Can you work these out from the model? Positions are in its coordinate system, mm. A direction names the side the tool comes from. Coordinates: 2 decimals unless noted, no trailing zeros. Loops run counter-clockwise (first coordinate to the right, second up) from the corner with the lowest first, then second, coordinate; pieces in that order, holes last. Notation, with made-up numbers: (42, 87.5) -> (54, 87.5) arc R14 ccw to (54, 96.5) -> close; hole circle Ø2 at (5.5, 39.25). An arc over 180 degrees is marked (long way). Put each result on its own line as item: value. Start each with the question number.
Item 1: Please list where these lines run through material, in increasing order: L1, parallel to Z at x = 25.09, y = 16.85; L2, parallel to Z at x = 8, y = 21; L3, parallel to X at y = 2, z = -4.5. Write a range as from..to.
Item 2: If we section it at C-C on x = 10.75: Please give me the cut outline in (y, z), plus the area to 3 significant figures.
Item 3: For faces 1 (the flat face through (23.9, 16, -6.2)), 2 (the flat face through (0, 8, -6)), 3 (the cylindrical face through (8.1, 24.5, -6.2)), which set-ups out of +Z, -Z, +X, -X, +Y, -Y let a thin tool reach every point of the face, with its end or its side?
Item 4: If we section it at D-D on z = -4.5: Please give me the cut outline in (x, y), plus the area to 3 significant figures.
Item 5: We'd pull the mould along Z, two halves only. Please class faces 4 (the cylindrical face through (-1.74, 17.27, -6.31)), 5 (the flat face through (27, 17, -5.862)), 6 (the flat face through (27.25, 17, -9)), 7 (the cylindrical face through (14.96, 28.23, -7.79)): pulls with the +Z half, pulls with the -Z half, needs draft (parallel to the pull), parting line crosses it, or undercut.
Item 6: Will these pins go through, and if not, where does the flat tip stop? P1, Ø1.5, axis at x = -3, z = -3.5, coming from the -Y side; P2, Ø3, axis at y = 5, z = -1.5, coming from the -X side; P3, Ø1.4, axis at x = 27, y = 17, coming from the -Z side.
Item 7: If we section it at B-B on y = 17: Please give me the cut outline in (x, z), plus the area to 3 significant figures.
Item 8: If we section it at A-A on x = -2.74: Please give me the cut outline in (y, z), plus the area to 3 significant figures.
```python
from build123d import *

# Parameters (mm, degrees)
SKETCH1_W           = 22.65
SKETCH1_H           = 12.25
BOSS_EXTRUDE1_DEPTH = 16
SKETCH2_W           = 32.15
SKETCH2_H           = 12.2
BOSS_EXTRUDE2_DEPTH = 2.5
SKETCH3_W           = 22.6
SKETCH3_H           = 12.2
BOSS_EXTRUDE3_DEPTH = 4
BOSS_EXTRUDE4_DEPTH = 4.15
SKETCH5_R           = 2.5
BOSS_EXTRUDE5_DEPTH = 3.2
CUT_EXTRUDE1_DEPTH  = 19.5


with BuildPart() as part:
    # Sketch1 → Boss-Extrude1 (new body)
    with BuildSketch(Plane(origin=(0, 0, 0), x_dir=(1, 0, 0), z_dir=(0, 1, 0))):
        with Locations((11.325, 6.125)):
            Rectangle(SKETCH1_W, SKETCH1_H)
    extrude(amount=BOSS_EXTRUDE1_DEPTH)

    # Sketch2 → Boss-Extrude2 (add)
    with BuildSketch(Plane(origin=(0, 16, 0), x_dir=(1, 0, 0), z_dir=(0, 1, 0))):
        with Locations((11.175, 6.1)):
            Rectangle(SKETCH2_W, SKETCH2_H)
    extrude(amount=BOSS_EXTRUDE2_DEPTH)

    # Sketch3 → Boss-Extrude3 (add)
    with BuildSketch(Plane(origin=(0, 18.5, 0), x_dir=(1, 0, 0), z_dir=(0, 1, 0))):
        with Locations((11.3, 6.1)):
            Rectangle(SKETCH3_W, SKETCH3_H)
    extrude(amount=BOSS_EXTRUDE3_DEPTH)

    # Sketch4 → Boss-Extrude4 (add)
    with BuildSketch(Plane(origin=(0, 22.5, 0), x_dir=(1, 0, 0), z_dir=(0, 1, 0))):
        with BuildLine():
            ThreePointArc((11.66557377, 3.61318986), (22.6, 6.1), (11.66557377, 8.58681014))
            ThreePointArc((11.66557377, 8.58681014), (8.1, 6.1), (11.66557377, 3.61318986))
        make_face()
    extrude(amount=BOSS_EXTRUDE4_DEPTH)

    # Sketch5 → Boss-Extrude5 (add)
    with BuildSketch(Plane(origin=(0, 26.65, 0), x_dir=(1, 0, 0), z_dir=(0, 1, 0))):
        with Locations((16.8, 6.1)):
            Circle(SKETCH5_R)
    extrude(amount=BOSS_EXTRUDE5_DEPTH)

    # Sketch6 → Cut-Extrude1 (cut, through all)
    with BuildSketch(Plane(origin=(0, 18.5, 0), x_dir=(1, 0, 0), z_dir=(0, 1, 0))):
        with BuildLine():
            Line((-3.615686095, 5.766143081), (-4.9, 5.766143081))
            Line((-4.9, 5.766143081), (-4.9, 6.689056169))
            Line((-4.9, 6.689056169), (-3.63798195, 6.689056169))
            ThreePointArc((-3.63798195, 6.689056169), (-1.74029168, 6.273174961), (-3.615686095, 5.766143081))
        make_face()
        with BuildLine():
            Line((26.012019834, 5.861881235), (27.25, 5.861881235))
            Line((27.25, 5.861881235), (27.25, 6.689056169))
            Line((27.25, 6.689056169), (25.98798195, 6.689056169))
            ThreePointArc((25.98798195, 6.689056169), (24.090421981, 6.219975921), (26.012019834, 5.861881235))
        make_face()
    extrude(amount=-CUT_EXTRUDE1_DEPTH, mode=Mode.SUBTRACT)


solid = part.part
```
Solutions:
1. L1: -12.2..-7.25, -5.25..0
1. L2: -12.2..0
1. L3: 0..22.65
2. outline: (0, -12.25) -> (16, -12.25) -> (16, -12.2) -> (22.5, -12.2) -> (22.5, -8.75) -> (26.65, -8.75) -> (26.65, -3.45) -> (22.5, -3.45) -> (22.5, 0) -> (0, 0) -> close
2. area: 297 mm^2
3. face 1: +Z, -Z, +X, -Y
3. face 2: +Z, -Z, -X, -Y
3. face 3: +Y
4. outline: (-4.9, 16) -> (0, 16) -> (0, 0) -> (22.65, 0) -> (22.65, 16) -> (27.25, 16) -> (27.25, 18.5) -> (22.6, 18.5) -> (22.6, 22.5) -> (22.37, 22.5) -> (22.37, 26.65) -> (18.72, 26.65) -> (18.72, 29.85) -> (14.88, 29.85) -> (14.88, 26.65) -> (8.64, 26.65) -> (8.64, 22.5) -> (0, 22.5) -> (0, 18.5) -> (-4.9, 18.5) -> close
4. area: 602 mm^2
5. face 4: undercut
5. face 5: undercut
5. face 6: needs draft
5. face 7: parting line crosses it
6. P1: y = 16
6. P2: x = 0
6. P3: z = -12.2
7. outline: (-4.9, -12.2) -> (27.25, -12.2) -> (27.25, -6.69) -> (25.99, -6.69) arc R1 cw (long way) to (26.01, -5.86) -> (27.25, -5.86) -> (27.25, 0) -> (-4.9, 0) -> (-4.9, -5.77) -> (-3.62, -5.77) arc R1 cw (long way) to (-3.64, -6.69) -> (-4.9, -6.69) -> close
7. area: 384 mm^2
8. outline: (16, -12.2) -> (18.5, -12.2) -> (18.5, -7.25) -> (16, -7.25) -> close; (16, -5.25) -> (18.5, -5.25) -> (18.5, 0) -> (16, 0) -> close
8. area: 25.5 mm^2
